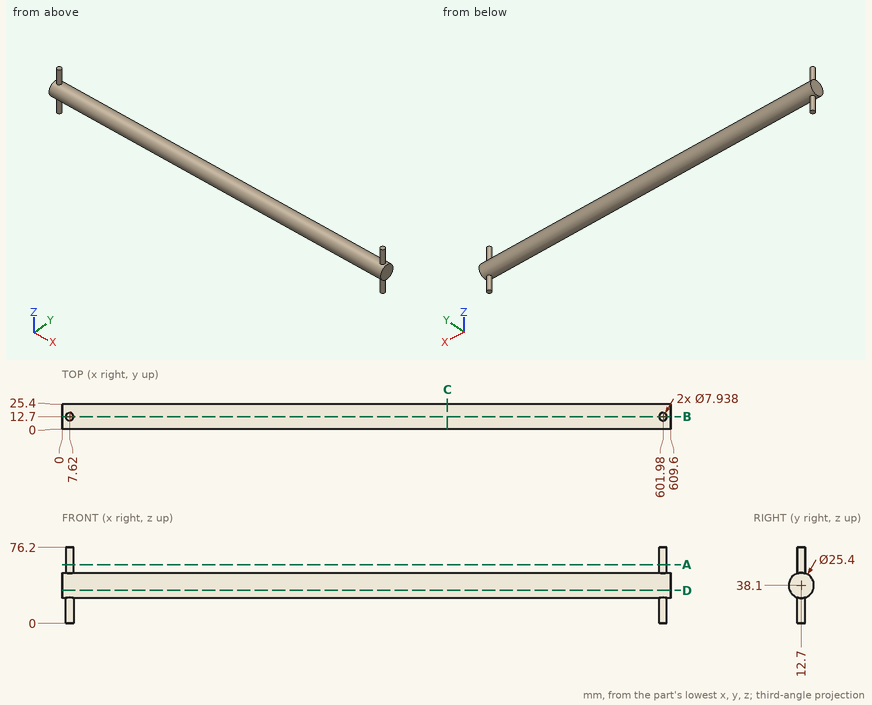
Verification items for this drawing (mm, ordinates from the low corner). Give positions to 0.01 mm unless a question says otherwise; leave off trailing zeros. Loops run counter-clockwise (first coordinate to the right, second up) from the corner with the lowest first, then second, coordinate; pieces in that order, holes last. Notation, with made-up numbers: M -33.75,17 L 0.25,17 A14 cw 0.25,37 Z; hole C -8.5,-30 d9. An arc over 180 degrees is marked long. Write item = value, one per line.
(1) Sectioned sample at D-D, the plane z = 33. Record the cut outline in (x, y).
Answer below:
outline = M 0,1.07 L 609.6,1.07 L 609.6,24.33 L 0,24.33 Z
(2) Material ranges on line 1 (Z direction, x = 340, y = 2.5) (1 decimal); line 2 (Y direction, x = 419, z = 36.5); line 3 (Y direction, x = 89.5, z = 33), recorded low to high. Write a range as [from, to].
Answer below:
line_1 = [30.5, 45.7]
line_2 = [0.1, 25.3]
line_3 = [1.07, 24.33]
(3) Sectioned sample at C-C, the plane x = 386. Record the cut outline in (y, z).
Answer below:
outline = C 12.7,38.1 d25.4
(4) Sectioned sample at B-B, the plane y = 12.7. Record the cut outline in (x, z).
Answer below:
outline = M 0,25.4 L 3.65,25.4 L 3.65,0 L 11.59,0 L 11.59,25.4 L 598.01,25.4 L 598.01,0 L 605.95,0 L 605.95,25.4 L 609.6,25.4 L 609.6,50.8 L 605.95,50.8 L 605.95,76.2 L 598.01,76.2 L 598.01,50.8 L 11.59,50.8 L 11.59,76.2 L 3.65,76.2 L 3.65,50.8 L 0,50.8 Z
(5) Sectioned sample at A-A, the plane z = 59. Record the cut outline in (x, y).
Answer below:
outline = C 7.62,12.7 d7.94; C 601.98,12.7 d7.94
(6) Gauge pin test, flat ends, axial feed: pin 1 Ø2 at (x, y) = (130, 23) entering from +Z; pin 2 Ø1.5 at (x, y) = (165, 3.5) entering from -Z; pin 3 Ø2 at (x, y) = (192, 12.5) entering from -Z. Record the tip position at first contact, or that the pin passes through.
Answer below:
pin_1 = 46.75
pin_2 = 28.62
pin_3 = 25.4
